Read the model definition and answer for the solid it produces. Units are mm, in the model's axes. Face numbers are marked on the shaded views. A direction names the side the tool comes from. Coordinates: 2 decimals unless noted, no trailing zeros. Loops run counter-clockwise (first coordinate to the right, second up) from the corner with the lowest first, then second, coordinate; pieces in that order, holes last. Notation, with made-up numbers: (-33.75, 6.5) - (1.25, 6.5) arc R11 ccw to (1.25, 26.5) - close; hole circle Ø7 at (83, 61). An arc over 180 degrees is marked (long way). Use one line per item in the form item = value. Start each with the question number.
1) The mould has two halves that part along X. Classify the marked faces 1, 2, 3 and 4: released by +X, released by -X, zero draft, split by the parting line, or undercut.
2) A cutting plane is placed at A-A (x = 20). Give the vertices of the cut face in (y, z).
3) A cutting plane is placed at B-B (z = -7.5). Give the vertices of the cut face in (x, y), and give its area (3 significant figures).
4) A cutting plane is placed at C-C (x = 0). Give the vertices of the cut face in (y, z).
5) Consider line 1 (X direction, y = 3.05, z = 0); line 2 (Z direction, x = -8, y = 3.65); line 3 (X direction, y = 2, z = 20). Determine where each line is inside the solid, lowest interval first.
6) A cutting plane is placed at D-D (y = 4.85). Give the vertices of the cut face in (x, z), and give its area (3 significant figures).
7) Which of the six approach directions +Z, -Z, +X, -X, +Y, -Y give full straight-line access (tool end or side, diameter ignored) to the marked faces 5, 6, 7, 8 and 9?
8) Each of these flat-tipped pins is pushed along its axis until it touches: P1, Ø3, axis at y = 4, z = -14, coming from the -X side; P2, Ø1.8, axis at y = 4.5, z = 13, coming from the +X side; P3, Ø1, axis at x = -4, y = 2, coming from the +Z side; P4, Ø6, axis at x = 0, z = -20, coming from the +Y side (1 decimal). Where does it stop, or does it pass through?
from build123d import *

# Parameters (mm, degrees)
SKETCH1_R           = 3.25
BOSS_EXTRUDE1_DEPTH = 6


with BuildPart() as part:
    # Sketch1 → Boss-Extrude1 (new body)
    with BuildSketch(Plane(origin=(0, 0, 0), x_dir=(1, 0, 0), z_dir=(0, 1, 0))):
        with BuildLine():
            Line((-24, -4.668943148), (-24, -24))
            Line((-24, -24), (-4.802343178, -24))
            ThreePointArc((-4.802343178, -24), (0, -26.25), (4.802343178, -24))
            Line((4.802343178, -24), (24, -24))
            Line((24, -24), (24, -4.802343178))
            ThreePointArc((24, -4.802343178), (26.25, 0), (24, 4.802343178))
            Line((24, 4.802343178), (24, 24))
            Line((24, 24), (4.802343178, 24))
            ThreePointArc((4.802343178, 24), (0, 26.25), (-4.802343178, 24))
            Line((-4.802343178, 24), (-24, 24))
            Line((-24, 24), (-24, 5.04363247))
            ThreePointArc((-24, 5.04363247), (-26.315667945, 0.187344661), (-24, -4.668943148))
        make_face()
        with Locations(Location((-20.065667945, 0.187344661, 0), (0, 0, 270))):
            Circle(SKETCH1_R, mode=Mode.SUBTRACT)
        with Locations(Location((0, 20, 0), (0, 0, 270))):
            Circle(SKETCH1_R, mode=Mode.SUBTRACT)
        with Locations(Location((20, 0, 0), (0, 0, 270))):
            Circle(SKETCH1_R, mode=Mode.SUBTRACT)
        with Locations(Location((0, -20, 0), (0, 0, 270))):
            Circle(SKETCH1_R, mode=Mode.SUBTRACT)
        with BuildLine():
            Line((-16, 16), (-4.802343178, 16))
            ThreePointArc((-4.802343178, 16), (0, 13.75), (4.802343178, 16))
            Line((4.802343178, 16), (16, 16))
            Line((16, 16), (16, 4.802343178))
            ThreePointArc((16, 4.802343178), (13.75, 0), (16, -4.802343178))
            Line((16, -4.802343178), (16, -16))
            Line((16, -16), (4.802343178, -16))
            ThreePointArc((4.802343178, -16), (0, -13.75), (-4.802343178, -16))
            Line((-4.802343178, -16), (-16, -16))
            Line((-16, -16), (-16, -4.559532645))
            ThreePointArc((-16, -4.559532645), (-13.815667945, 0.187344661), (-16, 4.934221967))
            Line((-16, 4.934221967), (-16, 16))
        make_face(mode=Mode.SUBTRACT)
    extrude(amount=BOSS_EXTRUDE1_DEPTH)


solid = part.part
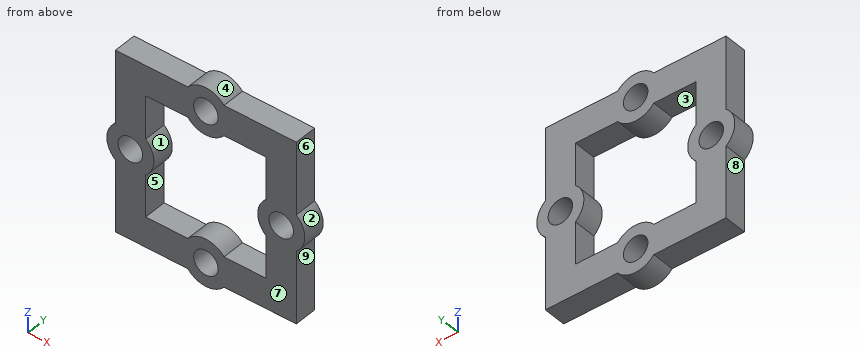
Found:
q1.face_1 = undercut
q1.face_2 = released by +X
q1.face_3 = undercut
q1.face_4 = split by the parting line
q2.outline = (0, -24) - (6, -24) - (6, -3.25) - (0, -3.25) - close; (0, 3.25) - (6, 3.25) - (6, 24) - (0, 24) - close
q3.outline = (-24, 0) - (-16, 0) - (-16, 6) - (-24, 6) - close; (16, 0) - (24, 0) - (24, 6) - (16, 6) - close
q3.area = 96.0 mm^2
q4.outline = (0, -26.25) - (6, -26.25) - (6, -23.25) - (0, -23.25) - close; (0, -16.75) - (6, -16.75) - (6, -13.75) - (0, -13.75) - close; (0, 13.75) - (6, 13.75) - (6, 16.75) - (0, 16.75) - close; (0, 23.25) - (6, 23.25) - (6, 26.25) - (0, 26.25) - close
q5.line_1 = -26.31 to -23.31, -16.82 to -13.82, 13.75 to 16.75, 23.25 to 26.25
q5.line_2 = -24 to -16, 16 to 24
q5.line_3 = -24 to -3.25, 3.25 to 24
q6.outline = (-24, -24) - (-4.8, -24) arc R6.25 ccw to (4.8, -24) - (24, -24) - (24, -4.8) arc R6.25 ccw to (24, 4.8) - (24, 24) - (4.8, 24) arc R6.25 ccw to (-4.8, 24) - (-24, 24) - (-24, 4.67) arc R6.25 ccw to (-24, -5.04) - close; hole circle Ø6.5 at (-20.07, -0.19); hole (-16, -16) - (-4.8, -16) arc R6.25 cw to (4.8, -16) - (16, -16) - (16, -4.8) arc R6.25 cw to (16, 4.8) - (16, 16) - (4.8, 16) arc R6.25 cw to (-4.8, 16) - (-16, 16) - (-16, 4.56) arc R6.25 cw to (-16, -4.93) - close; hole circle Ø6.5 at (0, -20); hole circle Ø6.5 at (0, 20); hole circle Ø6.5 at (20, 0)
q6.area = 1,270 mm^2
q7.face_5 = +Y, -Y
q7.face_6 = +Z, +X, +Y, -Y
q7.face_7 = +Z, -Z, +X, -X, -Y
q7.face_8 = -Z, -X, +Y, -Y
q7.face_9 = -Z, +X, +Y, -Y
q8.P1 = -24
q8.P2 = 24
q8.P3 = 25.18
q8.P4 = through
